```python
from build123d import *

# Parameters (mm, degrees)
FILLET1_R    = 0.1
SKETCH3_W    = 0.74
SKETCH3_H    = 2.6
SKETCH4_W    = 0.74
SKETCH4_H    = 1.104255426
RECPAT_COUNT = 2
RECPAT_ANGLE = 90


with BuildPart() as part:
    # BodySke → Base-Revolve (revolve)
    with BuildSketch(Plane.XY):
        with BuildLine():
            Line((2.1, 1.25), (2.1, 2.5))
            Line((2.1, 2.5), (0.99500416, 2.5))
            ThreePointArc((0.99500416, 2.5), (0.88781572, 2.474733878), (0.803195915, 2.404255319))
            ThreePointArc((0.803195915, 2.404255319), (0.206109099, 1.267435138), (0, 0))
            Line((0, 0), (10.1, 0))
            Line((10.1, 0), (10.1, 1.25))
            Line((10.1, 1.25), (2.1, 1.25))
        make_face()
    revolve(axis=Axis((-25.4, 0, 0), (1, 0, 0)))

    # Fillet1
    fillet1_edges = [part.edges().sort_by_distance(p)[0] for p in [
        (2.1, -1.25, 0),
    ]]
    fillet(fillet1_edges, radius=FILLET1_R)

    # Sketch3 → Recess section 0
    with BuildSketch(Plane(origin=(0, 0, 0), x_dir=(0, 0, -1), z_dir=(1, 0, 0))):
        Rectangle(SKETCH3_W, SKETCH3_H)
    # Sketch4 → Recess section 1
    with BuildSketch(Plane(origin=(1.5, 0, 0), x_dir=(0, 0, -1), z_dir=(1, 0, 0))):
        Rectangle(SKETCH4_W, SKETCH4_H)
    recess = loft(mode=Mode.SUBTRACT)

    # RecPat: Recess ×2 about axis
    recpat_axis = Axis((0, 0, 0), (1, 0, 0))
    for i in range(1, RECPAT_COUNT):
        add(recess.rotate(recpat_axis, i * RECPAT_ANGLE / (RECPAT_COUNT - 1)), mode=Mode.SUBTRACT)

    # RecCorSke → RecessCore (revolve, cut)
    with BuildSketch(Plane.XY):
        Polygon((0, 0), (0, 0.660890218), (1.5, 0.556), (1.680655351, 0), align=None)
    revolve(axis=Axis((-3.175, 0, 0), (1, 0, 0)), mode=Mode.SUBTRACT)


solid = part.part
```
Model file for the job. Use its own axes, mm. A direction names the side the tool comes from. Round coordinates to 2 decimals unless told otherwise and drop trailing zeros. Write each loop counter-clockwise with the first axis right and the second up, starting at its lowest first coordinate (ties: lowest second). Pieces come first, ordered by that corner, then holes. Notation, with made-up numbers: (18, 25) -> (74, 25) arc R27 ccw to (74, 53) -> close; hole circle Ø7 at (-30.75, -4). An arc over 180 degrees is marked (long way). Answer as CSV lines item,"result".
1. Pin check, flat tips, straight feed: pin 1 Ø1.5 at (x, y) = (3.5, 1.5) entering from +Z; pin 2 Ø3 at (x, z) = (7, -1.5) entering from -Y; pin 3 Ø1 at (x, z) = (2, -1) entering from +Y. Stop position of each tip, or through.
Resolved:
pin 1,"z = 1"
pin 2,"y = -1.25"
pin 3,"y = 2.45"
2. Drill centre lines: line 1 (X direction, y = 1.75, z = -0.3); line 2 (Y direction, x = 0.75, z = -1.9); line 3 (X direction, y = -0.2, z = -0.9). Where is each one in solid material? Low to high.
Resolved:
line 1,"0.42 to 2.1"
line 2,"-1.35 to 1.35"
line 3,"0.8 to 10.1"
3. Mould opens along Y. For faces 1 (the face through (10.1, 0, 0)), 2 (the face through (6.09, -0.27, -1.22)), 3 (the face through (1.67, 0.03, 0.01)) say: +Y half, -Y half, draft (parallel to the pull), parting line (faces both ways), or undercut.
Resolved:
face 1,"draft"
face 2,"parting line"
face 3,"undercut"
4. Slice it at B-B, the plane x = 3.25. List the corners of the cut face in (y, z), plus the area to 3 significant figures.
Resolved:
outline,"circle Ø2.5 at (0, 0)"
area,"4.91 mm²"
5. Slice it at A-A, the plane x = 2. List the corners of the cut face in (y, z).
Resolved:
outline,"circle Ø5 at (0, 0)"
6. Tool access for faces 4 (the face through (1.54, -0.54, -2.44)), 5 (the face through (2.1, -1.1, -1.1)): list every direction of +Z, -Z, +X, -X, +Y, -Y with a clear straight run to the whole face (end or side of a thin tool).
Resolved:
face 4,"+X, -X"
face 5,"+X"
